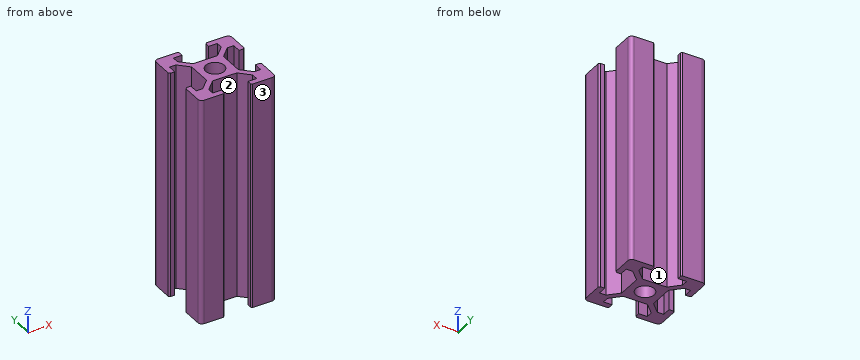
Autodesk Fusion 360 part; units mm, degrees
sketch "Sketch1" plane through (0, 0, 0) normal (0, 0, 1) x (1, 0, 0)
  line L0 (0, 1) -> (0, 6.1503)
  line L1 (1, 0) -> (6.15, 0)
  line L2 (0.3536, 6.5038) -> (1.5038, 6.5038)
  line L3 (1.5038, 6.5038) -> (1.5038, 4.2038)
  line L4 (1.5038, 4.2038) -> (3.2139, 4.2038)
  line L5 (3.2139, 4.2038) -> (5.804, 6.7939)
  line L6 (6.5036, 0.3536) -> (6.5036, 1.5036)
  line L7 (6.5036, 1.5036) -> (4.2036, 1.5036)
  line L8 (4.2036, 1.5036) -> (4.2036, 3.2136)
  line L9 (4.2036, 3.2136) -> (6.7937, 5.8037)
  line L10 (0, 6.1503) -> (0.3536, 6.5038)
  line L11 (6.15, 0) -> (6.5036, 0.3536)
  circle A0 centre (10, 10) radius 2.45
  line L12 (10, 10) -> (0, 0) construction
  line L13 (0, 19) -> (0, 13.85)
  line L14 (1, 20) -> (6.15, 20)
  line L15 (0, 13.85) -> (0.3536, 13.4964)
  line L16 (0, 13.85) -> (0.5, 13.85) construction
  line L17 (0.3536, 13.4964) -> (1.5036, 13.4964)
  line L18 (1.5036, 13.4964) -> (1.5036, 15.7964)
  line L19 (0, 20) -> (10, 10) construction
  line L20 (5.804, 6.7939) -> (5.804, 13.2061)
  line L21 (5.804, 13.2061) -> (3.2139, 15.7962)
  line L22 (1.5036, 15.7964) -> (3.2139, 15.7962)
  line L23 (6.15, 20) -> (6.5036, 19.6464)
  line L24 (6.15, 20) -> (6.65, 20) construction
  line L25 (6.5036, 19.6464) -> (6.5036, 18.4964)
  line L26 (6.5036, 18.4964) -> (4.2036, 18.4964)
  line L27 (4.2036, 18.4964) -> (4.2036, 16.7864)
  line L28 (4.2036, 16.7864) -> (6.7937, 14.1963)
  line L29 (10, 10) -> (20, 20) construction
  line L30 (10, 10) -> (20, 0) construction
  line L31 (19, 20) -> (13.85, 20)
  line L32 (20, 19) -> (20, 13.85)
  line L33 (13.85, 20) -> (13.4964, 19.6464)
  line L34 (13.85, 20) -> (14.35, 20) construction
  line L35 (13.4964, 19.6464) -> (13.4964, 18.4964)
  line L36 (20, 13.85) -> (19.6464, 13.4964)
  line L37 (20, 13.85) -> (20.5, 13.85) construction
  line L38 (19.6464, 13.4964) -> (18.4964, 13.4964)
  line L39 (13.4964, 18.4964) -> (15.7964, 18.4964)
  line L40 (18.4964, 13.4964) -> (18.4964, 15.7964)
  line L41 (15.7964, 18.4964) -> (15.7964, 16.7864)
  line L42 (15.7964, 16.7864) -> (13.2064, 14.1963)
  line L43 (13.2064, 14.1963) -> (6.7937, 14.1963)
  line L44 (18.4964, 15.7964) -> (16.7864, 15.7964)
  line L45 (16.7864, 15.7964) -> (14.1963, 13.2063)
  line L46 (19, 0) -> (13.85, 0)
  line L47 (20, 1) -> (20, 6.15)
  line L48 (13.85, 0) -> (13.4964, 0.3536)
  line L49 (13.85, 0) -> (14.35, 0) construction
  line L50 (13.4964, 0.3536) -> (13.4964, 1.5036)
  line L51 (13.4964, 1.5036) -> (15.7964, 1.5036)
  line L52 (15.7964, 1.5036) -> (15.7964, 3.2136)
  line L53 (15.7964, 3.2136) -> (13.2063, 5.8037)
  line L54 (6.7937, 5.8037) -> (13.2063, 5.8037)
  line L55 (20, 6.15) -> (19.6464, 6.5036)
  line L56 (20, 6.15) -> (20.5, 6.15) construction
  line L57 (19.6464, 6.5036) -> (18.4964, 6.5036)
  line L58 (18.4964, 6.5036) -> (18.4964, 4.2036)
  line L59 (18.4964, 4.2036) -> (16.7864, 4.2036)
  line L60 (16.7864, 4.2036) -> (14.1963, 6.7937)
  line L61 (14.1963, 6.7937) -> (14.1963, 13.2063)
  arc A1 (0, 1) -> (1, 0) centre (1, 1) ccw
  arc A2 (1, 20) -> (0, 19) centre (1, 19) ccw
  arc A3 (20, 19) -> (19, 20) centre (19, 19) ccw
  arc A4 (19, 0) -> (20, 1) centre (19, 1) ccw
  dimension "d9" = 2.3
  dimension "d11" = 3.663
  dimension "d13" = 2.3
  dimension "d17" = 135
  dimension "d18" = 135
  dimension "d19" = 135
  dimension "d20" = 6.1503
  dimension "d21" = 1.1503
  dimension "d22" = 0.5
  dimension "d23" = 135
  dimension "d24" = 0.5
  dimension "d25" = 6.15
  dimension "d26" = 1.15
  dimension "d27" = 4.9
  dimension "d28" = 10
  dimension "d29" = 10
  dimension "d30" = 1.4
  dimension "d31" = 0.7
  dimension "d32" = 6.15
  dimension "d33" = 20
  dimension "d34" = 6.15
  dimension "d35" = 45
  dimension "d36" = 0.5
  dimension "d37" = 1.15
  dimension "d38" = 2.3
  dimension "d40" = 3.663
  dimension "d41" = 0.7
  dimension "d42" = 0.5
  dimension "d43" = 45
  dimension "d44" = 1.15
  dimension "d45" = 2.3
  dimension "d47" = 3.663
  dimension "d48" = 0.7
  dimension "d49" = 6.15
  dimension "d50" = 6.15
  dimension "d51" = 135
  dimension "d52" = 0.5
  dimension "d53" = 1.15
  dimension "d54" = 20
  dimension "d55" = 135
  dimension "d56" = 0.5
  dimension "d57" = 1.15
  dimension "d58" = 2.3
  dimension "d59" = 2.3
  dimension "d61" = 0.7
  dimension "d63" = 3.663
  dimension "d64" = 0.7
  dimension "d65" = 6.15
  dimension "d66" = 6.15
  dimension "d67" = 135
  dimension "d68" = 0.5
  dimension "d69" = 20
  dimension "d70" = 1.15
  dimension "d71" = 2.3
  dimension "d73" = 0.7
  dimension "d74" = 135
  dimension "d75" = 0.5
  dimension "d76" = 1.15
  dimension "d77" = 2.3
  dimension "d78" = 1.71
  dimension "d79" = 1
  dimension "d80" = 1
  dimension "d81" = 1
  dimension "d82" = 1
  dimension "d83" = 1
  dimension "d84" = 1
extrude "Extrude1" add sketch "Sketch1" along normal blind 60
Build history of the part. All positions in model axes, mm. Face numbers are marked on the shaded views. Give positions to 0.01 mm unless a question says otherwise; leave off trailing zeros. Loops run counter-clockwise (first coordinate to the right, second up) from the corner with the lowest first, then second, coordinate; pieces in that order, holes last. Notation, with made-up numbers: (-36, -7.75) -> (-28, -7.75) arc R18 cw to (-28, 5.25) -> close; hole circle Ø7 at (50, 16.5). An arc over 180 degrees is marked (long way). One line per question, with ' | ' between items. Start each with the question number.
1) Cut at A-A (y = 10). Give the cut face in (x, z).
2) Two-plate mould, pull along X, no slides. Class the marked faces 1, 2 and 3: released by +X, released by -X, zero draft, split by the parting line, or undercut.
3) Probe L1, parallel to X at y = 4.5, z = 24; L2, parallel to X at y = 5.25, z = 23. List the from-to ranges inside material, lowest first.
4) Cut at C-C (x = 4.75). Give the cut face in (y, z).
5) Pin check, flat tips, straight feed: pin 1 (2 mm diameter, centred on x = 15.5, y = 8.5, fed in from +Z); pin 2 (3 mm diameter, centred on x = 9.5, z = 27.5, fed in from +Y); pin 3 (0.6 mm diameter, centred on x = 0.5, z = 35.5, fed in from +Y); pin 4 (2 mm diameter, centred on x = 9.5, z = 41.5, fed in from -Y). Stop position of each tip, or through.
Return value:
1) outline: (5.8, 0) -> (7.55, 0) -> (7.55, 60) -> (5.8, 60) -> close; (12.45, 0) -> (14.2, 0) -> (14.2, 60) -> (12.45, 60) -> close
2) face 1: undercut | face 2: undercut | face 3: zero draft
3) L1: 0 to 1.5, 3.51 to 5.49, 14.51 to 16.49, 18.5 to 20 | L2: 0 to 1.5, 4.26 to 6.24, 13.76 to 15.74, 18.5 to 20
4) outline: (0, 0) -> (1.5, 0) -> (1.5, 60) -> (0, 60) -> close; (3.76, 0) -> (5.74, 0) -> (5.74, 60) -> (3.76, 60) -> close; (14.26, 0) -> (16.24, 0) -> (16.24, 60) -> (14.26, 60) -> close; (18.5, 0) -> (20, 0) -> (20, 60) -> (18.5, 60) -> close
5) pin 1: through | pin 2: y = 14.2 | pin 3: y = 19.98 | pin 4: y = 5.8
